CAD build for the part. Positions are in the model's coordinates, mm. A direction names the side the tool comes from. Round coordinates to 2 decimals unless told otherwise and drop trailing zeros. Write each loop counter-clockwise with the first axis right and the second up, starting at its lowest first coordinate (ties: lowest second). Pieces come first, ordered by that corner, then holes. Notation, with made-up numbers: (6, 50.25) - (42, 50.25) arc R27 cw to (42, 76.25) - close; hole circle Ø3 at (-28, -10). An arc over 180 degrees is marked (long way). Answer in a Markdown table with one row per item.
```python
from build123d import *

# Parameters (mm, degrees)
PAD_DEPTH       = 31
CHAMFER_SIZE    = 4
SKETCH001_R     = 1.6
POCKET_DEPTH    = 18.6
SKETCH002_R     = 3.1
POCKET001_DEPTH = 14.6
POCKET002_DEPTH = 9.48
CHAMFER001_SIZE = 3


with BuildPart() as part:
    # Sketch → Pad (new body)
    with BuildSketch(Plane.XY):
        Polygon((-7.3, 1.64), (-7.3, 0), (9.74, 0), (11.3, 1.8), (11.3, 7.68), (9.74, 9.48), (7.3, 9.48), (7.3, 1.64), align=None)
    extrude(amount=PAD_DEPTH)

    # Chamfer
    chamfer_edges = [part.edges().sort_by_distance(p)[0] for p in [
        (7.3, 1.64, 15.5),
    ]]
    chamfer(chamfer_edges, length=CHAMFER_SIZE)

    # Sketch001 (on Face9 of Chamfer) → Pocket (cut)
    with BuildSketch(Plane.YZ.offset(11.3)):
        with Locations((4.74, 26.286)):
            Circle(SKETCH001_R)
        with Locations((4.74, 4.714)):
            Circle(SKETCH001_R)
        with BuildLine():
            ThreePointArc((6.34, 15.714), (4.74, 17.314), (3.14, 15.714))
            Line((3.14, 15.714), (3.14, 15.286))
            ThreePointArc((3.14, 15.286), (4.74, 13.686), (6.34, 15.286))
            Line((6.34, 15.286), (6.34, 15.714))
        make_face()
    extrude(amount=-POCKET_DEPTH, mode=Mode.SUBTRACT)

    # Sketch002 (on Face1 of Pocket) → Pocket001 (cut)
    with BuildSketch(Plane(origin=(7.3, 0, 0), x_dir=(0, -1, 0), z_dir=(-1, 0, 0))):
        with Locations((-4.74, 26.286)):
            Circle(SKETCH002_R)
        with Locations((-4.74, 4.714)):
            Circle(SKETCH002_R)
        with BuildLine():
            ThreePointArc((-1.64, 15.714), (-4.74, 18.814), (-7.84, 15.714))
            Line((-7.84, 15.714), (-7.84, 15.286))
            ThreePointArc((-7.84, 15.286), (-4.74, 12.186), (-1.64, 15.286))
            Line((-1.64, 15.286), (-1.64, 15.714))
        make_face()
    extrude(amount=POCKET001_DEPTH, mode=Mode.SUBTRACT)

    # Sketch003 (on Face33 of Pocket001) → Pocket002 (cut)
    with BuildSketch(Plane.XZ):
        with BuildLine():
            ThreePointArc((1.6, 27.4), (0, 29), (-1.6, 27.4))
            Line((-1.6, 27.4), (-1.6, 20.4))
            ThreePointArc((-1.6, 20.4), (0, 18.8), (1.6, 20.4))
            Line((1.6, 20.4), (1.6, 27.4))
        make_face()
        with BuildLine():
            ThreePointArc((1.6, 10.6), (0, 12.2), (-1.6, 10.6))
            Line((-1.6, 10.6), (-1.6, 3.6))
            ThreePointArc((-1.6, 3.6), (0, 2), (1.6, 3.6))
            Line((1.6, 3.6), (1.6, 10.6))
        make_face()
    extrude(amount=-POCKET002_DEPTH, mode=Mode.SUBTRACT)

    # Chamfer001
    chamfer001_edges = [part.edges().sort_by_distance(p)[0] for p in [
        (8.52, 9.48, 31),
        (8.52, 9.48, 0),
        (-7.3, 0.82, 0),
        (-7.3, 0.82, 31),
    ]]
    chamfer(chamfer001_edges, length=CHAMFER001_SIZE)


solid = part.part
```
Q1. Drill centre lines: line 1 (Z direction, x = 8.45, y = 4.74); line 2 (Z direction, x = 6.75, y = 4.25); line 3 (Z direction, x = 0.75, y = 1.5). Where is each one in solid material? Low to high.
Computed:
| item | result |
|---|---|
| line 1 | z = 0 to 3.11, 6.31 to 13.69, 17.31 to 24.69, 27.89 to 31 |
| line 2 | z = 0 to 1.65, 7.78 to 12.22, 18.78 to 23.22, 29.35 to 31 |
| line 3 | z = 0 to 2.19, 12.01 to 18.99, 28.81 to 31 |
Q2. Saw through at A-A on z = 9. List the corners of the cut face in (x, y), then the cut area to 3 significant figures.
Computed:
| item | result |
|---|---|
| outline | (-7.3, 0) - (-1.6, 0) - (-1.6, 1.64) - (-7.3, 1.64) - close; (1.6, 0) - (9.74, 0) - (11.3, 1.8) - (11.3, 7.68) - (9.74, 9.48) - (7.3, 9.48) - (7.3, 5.64) - (3.3, 1.64) - (1.6, 1.64) - close |
| area | 61.8 mm2 |
Q3. Saw through at B-B on x = 0. List the corners of the cut face in (y, z), then the cut area to 3 significant figures.
Computed:
| item | result |
|---|---|
| outline | (0, 0) - (1.64, 0) - (1.64, 2) - (0, 2) - close; (0, 12.2) - (1.64, 12.2) - (1.64, 18.8) - (0, 18.8) - close; (0, 29) - (1.64, 29) - (1.64, 31) - (0, 31) - close |
| area | 17.4 mm2 |
Q4. Flat gauge pins, fed straight in: pin 1 (3 mm diameter, centred on x = 4, z = 14.5, fed in from +Y); pin 2 (3.5 mm diameter, centred on y = 4.74, z = 4.714, fed in from -X); pin 3 (1 mm diameter, centred on x = 9.5, y = 7.5, fed in from +Z). Where does each tip first touch, or does it go through?
Computed:
| item | result |
|---|---|
| pin 1 | stops at y = 2.62 |
| pin 2 | stops at x = 7.3 |
| pin 3 | stops at z = 30.48 |
Q5. Pull direction X, two halves, no side cores. Call faces 1 (the cylindrical face through (0, 1, 2)), 2 (the flat face through (10.51, 0.89, 15.28)), 3 (the flat face through (5, 3, 31)), 4 (the cylindrical face through (0, 0.8, 18.8)): released by +X, released by -X, zero draft, split by the parting line, or undercut.
Computed:
| item | result |
|---|---|
| face 1 | undercut |
| face 2 | released by +X |
| face 3 | zero draft |
| face 4 | undercut |
Q6. Saw through at C-C on y = 4.74. List the corners of the cut face in (x, z).
Computed:
| item | result |
|---|---|
| outline | (6.4, 0) - (11.3, 0) - (11.3, 3.11) - (7.3, 3.11) - (7.3, 1.61) - (6.4, 1.61) - close; (6.4, 7.81) - (7.3, 7.81) - (7.3, 6.31) - (11.3, 6.31) - (11.3, 13.69) - (7.3, 13.69) - (7.3, 12.19) - (6.4, 12.19) - close; (6.4, 18.81) - (7.3, 18.81) - (7.3, 17.31) - (11.3, 17.31) - (11.3, 24.69) - (7.3, 24.69) - (7.3, 23.19) - (6.4, 23.19) - close; (6.4, 29.39) - (7.3, 29.39) - (7.3, 27.89) - (11.3, 27.89) - (11.3, 31) - (6.4, 31) - close |
Q7. Saw through at D-D on x = 9.25. List the corners of the cut face in (y, z), then the cut area to 3 significant figures.
Computed:
| item | result |
|---|---|
| outline | (0, 0) - (6.48, 0) - (9.48, 3) - (9.48, 28) - (6.48, 31) - (0, 31) - close; hole circle Ø3.2 at (4.74, 4.71); hole (3.14, 15.29) arc R1.6 ccw to (6.34, 15.29) - (6.34, 15.71) arc R1.6 ccw to (3.14, 15.71) - close; hole circle Ø3.2 at (4.74, 26.29) |
| area | 259 mm2 |
Q8. 3-axis set-ups, long thin cutter, end or side, ignore diameter. For faces 5 (the flat face through (9.33, 8, 1.52)), 6 (the flat face through (-1.6, 1, 24)): which of +Z, -Z, +X, -X, +Y, -Y reach the whole face in a straight line?
Computed:
| item | result |
|---|---|
| face 5 | -Z, +X, -X, +Y |
| face 6 | +Y, -Y |
